from build123d import *

# Parameters (mm, degrees)
EXTRUDE_1_DEPTH     = 20
CUT_EXTRUDE_1_DEPTH = 20
SKETCH_4_R          = 4.9
CUT_EXTRUDE_3_DEPTH = 3


with BuildPart() as part:
    # 草图1 → 凸台-拉伸1 (new body)
    with BuildSketch(Plane(origin=(0, 0, 0), x_dir=(1, 0, 0), z_dir=(0, 1, 0))):
        with BuildLine():
            Line((15, 0), (20, 0))
            Line((20, 0), (30, 0))
            Line((30, 0), (30, 6))
            Line((30, 6), (20, 6))
            Line((20, 6), (20, 20))
            ThreePointArc((20, 20), (0, 40), (-20, 20))
            Line((-20, 20), (-20, 6))
            Line((-20, 6), (-30, 6))
            Line((-30, 6), (-30, 0))
            Line((-30, 0), (-20, 0))
            Line((-20, 0), (-15, 0))
            Line((-15, 0), (-15, 20))
            ThreePointArc((-15, 20), (0, 35), (15, 20))
            Line((15, 20), (15, 0))
        make_face()
    extrude(amount=EXTRUDE_1_DEPTH)

    # 草图3 → 切除-拉伸1 (cut)
    with BuildSketch(Plane(origin=(0, 0, -6), x_dir=(-1, 0, 0), z_dir=(0, 0, -1))):
        with BuildLine():
            ThreePointArc((27.6, 10), (26.366900892, 12.211692102), (23.837244652, 12.325510697))
            Line((23.837244652, 12.325510697), (26.162755348, 7.674489303))
            ThreePointArc((26.162755348, 7.674489303), (27.211692102, 8.633099108), (27.6, 10))
        make_face()
        with BuildLine():
            Line((26.162755348, 7.674489303), (23.837244652, 12.325510697))
            ThreePointArc((23.837244652, 12.325510697), (22.674489303, 8.837244652), (26.162755348, 7.674489303))
        make_face()
        with BuildLine():
            ThreePointArc((-22.4, 10), (-23.633099108, 12.211692102), (-26.162755348, 12.325510697))
            Line((-26.162755348, 12.325510697), (-23.837244652, 7.674489303))
            ThreePointArc((-23.837244652, 7.674489303), (-22.788307898, 8.633099108), (-22.4, 10))
        make_face()
        with BuildLine():
            Line((-23.837244652, 7.674489303), (-26.162755348, 12.325510697))
            ThreePointArc((-26.162755348, 12.325510697), (-27.325510697, 8.837244652), (-23.837244652, 7.674489303))
        make_face()
    extrude(amount=-CUT_EXTRUDE_1_DEPTH, mode=Mode.SUBTRACT)

    # 草图4 → 切除-拉伸3 (cut)
    with BuildSketch(Plane(origin=(0, 0, -6), x_dir=(-1, 0, 0), z_dir=(0, 0, -1))):
        with Locations((-25, 10)):
            Circle(SKETCH_4_R)
        with Locations((25, 10)):
            Circle(SKETCH_4_R)
    extrude(amount=-CUT_EXTRUDE_3_DEPTH, mode=Mode.SUBTRACT)


solid = part.part
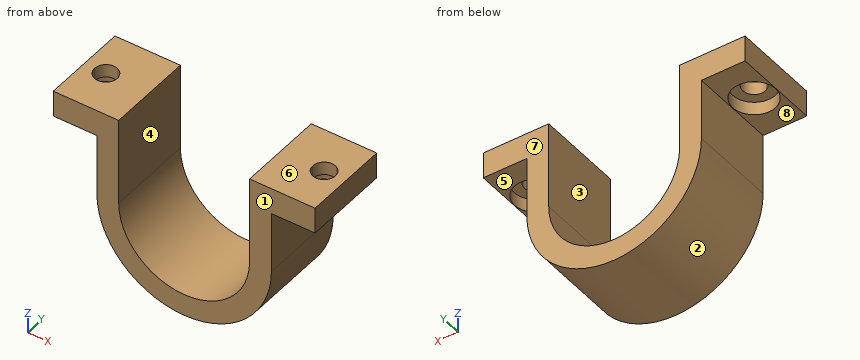
Build history of the part. All positions in model axes, mm. Face numbers are marked on the shaded views. A direction names the side the tool comes from. Give positions to 0.01 mm unless a question says otherwise; leave off trailing zeros. Write each loop counter-clockwise with the first axis right and the second up, starting at its lowest first coordinate (ties: lowest second). Pieces come first, ordered by that corner, then holes. Notation, with made-up numbers: (31, -39) - (86, -39) arc R10 ccw to (86, -32) - close; hole circle Ø10 at (80, -24.75). An arc over 180 degrees is marked (long way). Use one line per item in the form item = value. Start each with the question number.
1. 3-axis set-ups, long thin cutter, end or side, ignore diameter. For the marked faces 4, 5, 6, 7 and 8: which of +Z, -Z, +X, -X, +Y, -Y reach the whole face in a straight line?
2. Drop flat-ended pins along their axis: pin 1 Ø4 at (y, z) = (7, -10) entering from +X; pin 2 Ø3 at (y, z) = (7, -12.5) entering from -X; pin 3 Ø3 at (x, y) = (0.5, 3) entering from -Z. Give the stop position or say it passes through.
3. Two-plate mould, pull along X, no slides. Class the marked faces 1, 2 and 3: released by +X, released by -X, zero draft, split by the parting line, or undercut.
4. Band-saw the part on A-A on z = -13. Write the cut outline in (x, y).
5. Band-saw the part on D-D on z = -32. Write the cut outline in (x, y).
6. Probe line 1 (Y direction, x = -25, z = -4.15); line 2 (X direction, y = 19.25, z = -8.5); line 3 (Z direction, x = 21, y = 7.75). List the from-to ranges inside material, lowest first. Write a range as [from, to].
7. Band-saw the part on C-C on y = 2.25. Write the cut outline in (x, z).
8. Band-saw the part on B-B on x = 25. Write the cut outline in (y, z), plus the area to 3 significant figures.
Conclusion:
q1.face_4 = +Z, +Y, -Y
q1.face_5 = -Z, +X, +Y, -Y
q1.face_6 = +Z, +X, -X, +Y, -Y
q1.face_7 = +Z, -Z, +X, -X, +Y
q1.face_8 = -Z, -X, +Y, -Y
q2.pin_1 = 20
q2.pin_2 = -20
q2.pin_3 = -40
q3.face_1 = zero draft
q3.face_2 = split by the parting line
q3.face_3 = undercut
q4.outline = (-20, 0) - (-15, 0) - (-15, 20) - (-20, 20) - close; (15, 0) - (20, 0) - (20, 20) - (15, 20) - close
q5.outline = (-16, 0) - (-9, 0) - (-9, 20) - (-16, 20) - close; (9, 0) - (16, 0) - (16, 20) - (9, 20) - close
q6.line_1 = [0, 5.1], [14.9, 20]
q6.line_2 = [-20, -15], [15, 20]
q6.line_3 = [-3, 0]
q7.outline = (-30, -6) - (-20, -6) - (-20, -20) arc R20 ccw to (20, -20) - (20, -6) - (30, -6) - (30, 0) - (15, 0) - (15, -20) arc R15 cw to (-15, -20) - (-15, 0) - (-30, 0) - close
q8.outline = (0, -6) - (5.1, -6) - (5.1, -3) - (7.4, -3) - (7.4, 0) - (0, 0) - close; (12.6, -3) - (14.9, -3) - (14.9, -6) - (20, -6) - (20, 0) - (12.6, 0) - close
q8.area = 75.0 mm²
